The model under review builds one solid part; all positions refer to its coordinate system, in mm. Coordinates: 2 decimals unless noted, no trailing zeros. Order: outer loops, then holes, each group sorted by start corner. A loop starts at its lowest first (then second) coordinate and runs counter-clockwise, first axis right, second up. Notation, with made-up numbers: (60.25, -12.5) -> (77.25, -12.5) arc R32 cw to (77.25, 13.5) -> close; hole circle Ø6 at (-28, -3). An arc over 180 degrees is marked (long way). Use one line per item in the form item = value.
from build123d import *

# Parameters (mm, degrees)
BOSS_EXTRUDE1_DEPTH = 3.175
SKETCH2_R           = 3.175
CUT_EXTRUDE2_DEPTH  = 3.175
LPATTERN5_COUNT     = 3
LPATTERN5_PITCH     = 12.7
SKETCH7_R           = 3.175
CUT_EXTRUDE3_DEPTH  = 3.175
LPATTERN6_COUNT     = 3
LPATTERN6_PITCH     = 12.7


with BuildPart() as part:
    # Sketch1 → Boss-Extrude1 (new body)
    with BuildSketch(Plane(origin=(0, 0, 0), x_dir=(1, 0, 0), z_dir=(0, 1, 0))):
        Polygon((-25.4, 14.664696837), (0, 29.329393675), (25.4, 14.664696837), (56.694090512, -3.402954744), (43.994090512, -25.4), (0, 0), (-43.994090512, -25.4), (-56.694090512, -3.402954744), align=None)
    extrude(amount=BOSS_EXTRUDE1_DEPTH)

    # Sketch2 → Cut-Extrude2 (cut)
    with BuildSketch(Plane(origin=(0, 3.175, 0), x_dir=(1, 0, 0), z_dir=(0, 1, 0))):
        with Locations(Location((-39.345567884, -8.051477372, 0), (0, 0, 270))):
            Circle(SKETCH2_R)
    cut_extrude2 = extrude(amount=-CUT_EXTRUDE2_DEPTH, mode=Mode.SUBTRACT)

    # LPattern5: Cut-Extrude2 ×3
    with Locations(*[Vector(0.866025403784438, 0, -0.5000000000000012) * (i * LPATTERN5_PITCH) for i in range(1, LPATTERN5_COUNT)]):
        add(cut_extrude2, mode=Mode.SUBTRACT)

    # Sketch7 → Cut-Extrude3 (cut)
    with BuildSketch(Plane(origin=(0, 3.175, 0), x_dir=(1, 0, 0), z_dir=(0, 1, 0))):
        with Locations(Location((39.345567884, -8.051477372, 0), (0, 0, 270))):
            Circle(SKETCH7_R)
    cut_extrude3 = extrude(amount=-CUT_EXTRUDE3_DEPTH, mode=Mode.SUBTRACT)

    # LPattern6: Cut-Extrude3 ×3
    with Locations(*[Vector(-0.8660254037844382, 0, -0.500000000000001) * (i * LPATTERN6_PITCH) for i in range(1, LPATTERN6_COUNT)]):
        add(cut_extrude3, mode=Mode.SUBTRACT)


solid = part.part
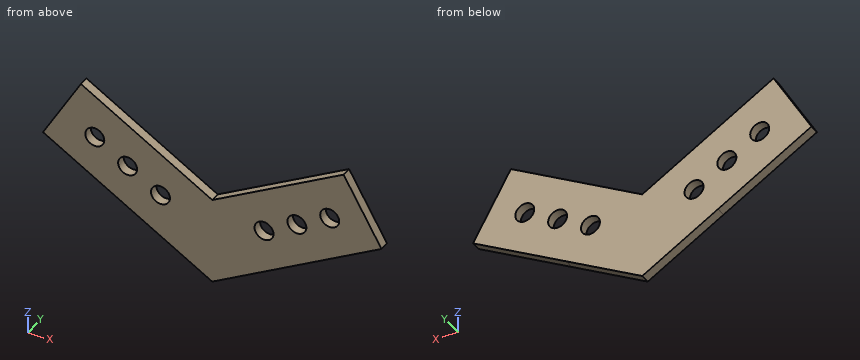
Item 1: Clearance check with a flat-ended pin moving along its axis: pin 1 (5.5 mm diameter, centred on x = -39.35, z = 8.05, fed in from -Y). State where the tip first meets the part, or that it passes through.
Results found:
pin_1 = through
Item 2: We need section D-D (z = 16.5). Write out the cut boundary in (x, y) (1 decimal).
Results found:
outline = (-49.1, 0) -> (-28.6, 0) -> (-28.6, 3.2) -> (-49.1, 3.2) -> close; (28.6, 0) -> (49.1, 0) -> (49.1, 3.2) -> (28.6, 3.2) -> close
Item 3: We need section B-B (y = 0.8). Write out the cut boundary in (x, z) (3 decimals).
Results found:
outline = (-56.694, 3.403) -> (0, -29.329) -> (56.694, 3.403) -> (43.994, 25.4) -> (0, 0) -> (-43.994, 25.4) -> close; hole circle Ø6.35 at (-39.346, 8.051); hole circle Ø6.35 at (-28.347, 1.701); hole circle Ø6.35 at (-17.349, -4.649); hole circle Ø6.35 at (17.349, -4.649); hole circle Ø6.35 at (28.347, 1.701); hole circle Ø6.35 at (39.346, 8.051)
Item 4: We need section C-C (z = -6.5). Write out the cut boundary in (x, y) (3 decimals).
Results found:
outline = (-39.542, 0) -> (-19.928, 0) -> (-19.928, 3.175) -> (-39.542, 3.175) -> close; (-14.769, 0) -> (14.769, 0) -> (14.769, 3.175) -> (-14.769, 3.175) -> close; (19.928, 0) -> (39.542, 0) -> (39.542, 3.175) -> (19.928, 3.175) -> close
Item 5: We need section A-A (z = 6.5). Write out the cut boundary in (x, y) (3 decimals).
Results found:
outline = (-54.906, 0) -> (-42.116, 0) -> (-42.116, 3.175) -> (-54.906, 3.175) -> close; (-36.575, 0) -> (-11.258, 0) -> (-11.258, 3.175) -> (-36.575, 3.175) -> close; (11.258, 0) -> (36.575, 0) -> (36.575, 3.175) -> (11.258, 3.175) -> close; (42.116, 0) -> (54.906, 0) -> (54.906, 3.175) -> (42.116, 3.175) -> close
Item 6: To check wall thickness, follow L1, parallel to X at y = 1.3, z = -3; L2, parallel to X at y = 1.6, z = -2.5; L3, parallel to Z at x = 40.5, y = 2.3. State the ranges of each line that lie inside material, in increasing order. Write a range as from..to.
Results found:
L1 = -45.6..-20.06, -14.64..14.64, 20.06..45.6
L2 = -46.47..-19.69, -15.01..15.01, 19.69..46.47
L3 = -5.95..5.09, 11.01..23.38
